For this review, take the finished solid that the model builds, in its own axes (mm). A direction names the side the tool comes from. Coordinates: 2 decimals unless noted, no trailing zeros. Loops run counter-clockwise (first coordinate to the right, second up) from the corner with the lowest first, then second, coordinate; pieces in that order, holes last. Notation, with made-up numbers: (7, 34) - (62, 34) arc R14 ccw to (62, 49) - close; hole circle Ø7 at (52.5, -26.5). An arc over 180 degrees is marked (long way). Answer as a JSON object with one key per item and string values. Group by question number.
Item 1: We need section B-B (z = 0). Give the boundary of the cut face in (x, y) (1 decimal), then the cut area to 3 significant figures.
Item 2: We need section C-C (y = 15.5). Give the boundary of the cut face in (x, z).
Item 3: To check wall thickness, follow line 1 (Y direction, x = 0, z = 5.4); line 2 (Z direction, x = -2.75, y = 20.75); line 3 (Y direction, x = 0.5, z = -5). State the ranges of each line that lie inside material, in increasing order.
Item 4: Tool access review of faces 1 (the flat face through (0, 6, -4.064)), 2 (the flat face through (3.086, 18, 0)), 3 (the flat face through (0, 18, -3.086)), 4 (the flat face through (-3.086, 18, 0)): name each direction out of +Z, -Z, +X, -X, +Y, -Y from which nothing blocks a thin tool from reaching the whole face with its end or side.
Item 5: Mouldability with a two-part tool opening along Z and no side actions: class faces 5 (the flat face through (0, 18, 3.086)), 6 (the flat face through (0, 6, 4.064)), 7 (the flat face through (0, 21.387, 0)), 8 (the conical face through (2.81, 21.23, -2.8)) as released by +Z, released by -Z, zero draft, split by the parting line, or undercut.
Item 6: We need section D-D (y = 10). Give the boundary of the cut face in (x, z), then the cut area to 3 significant figures.
Item 7: We need section A-A (x = 0). Give the boundary of the cut face in (y, z) (1 decimal), then the cut area to 3 significant figures.
Item 8: Clearance check with flat-ended pins moving along their axes: pin 1 (3 mm diameter, centred on x = -4, z = -1.5, fed in from -Y) (3 decimals); pin 2 (4 mm diameter, centred on x = -3.5, y = 7.5, fed in from +Z); pin 3 (1.9 mm diameter, centred on x = -0.5, y = 16.5, fed in from +Z). State where each tip first meets the part, or that it passes through.
from build123d import *

# Parameters (mm, degrees)
BASE_R                  = 6.9215
BASE_EXTRUDE_DEPTH      = 13.716
MALEDRIVE_R             = 6.0579
DRIVE_EXTRUDE_DEPTH     = 7.6708
SQDRIVE_SK_OUTSIDE_W    = 21.642
SQDRIVE_SK_OUTSIDE_H    = 21.642
SQDRIVE_SK_OUTSIDE_W_2  = 6.1722
SQDRIVE_SK_OUTSIDE_H_2  = 6.1722
DRIVE_SQCUT_DEPTH       = 7.6708
BASE_FILLET_TOP_R       = 0.762
PROFILE1_CUT_DEPTH      = 24.520406857
PROFILE1_CUT_DEPTH_BACK = 24.520406857
PROFILE1_CUTSK_W        = 8.128
PROFILE1_CUTSK_H        = 9.525
PROFILE2_CUT_DEPTH      = 24.520406857
PROFILE2_CUT_DEPTH_BACK = 24.520406857
PIN_CUT_DEPTH           = 24.520406916
PIN_CUT_DEPTH_BACK      = 24.520406916
PIN_CUTSK_R             = 1.778


with BuildPart() as part:
    # Base → Base-Extrude (new body)
    with BuildSketch(Plane(origin=(0, 0, 0), x_dir=(1, 0, 0), z_dir=(0, 1, 0))):
        with Locations(Location((0, 0, 0), (0, 0, 270))):
            Circle(BASE_R)
    extrude(amount=BASE_EXTRUDE_DEPTH)

    # MaleDrive → Drive-Extrude (add)
    with BuildSketch(Plane(origin=(0, 13.716, 0), x_dir=(1, 0, 0), z_dir=(0, 1, 0))):
        with Locations(Location((0, 0, 0), (0, 0, 270))):
            Circle(MALEDRIVE_R)
    extrude(amount=DRIVE_EXTRUDE_DEPTH)

    # Drive-ChamCut → DriveEnd-Chamfer (revolve, cut)
    with BuildSketch(Plane.XY, mode=Mode.PRIVATE) as driveend_chamfer_sk:
        Polygon((-3.81, 21.3868), (-5.4229, 19.7739), (-5.4229, 21.3868), align=None)
    revolve(driveend_chamfer_sk.sketch.rotate(Axis((0, 0, 0), (0, 1, 0)), 270), axis=Axis((0, 0, 0), (0, 1, 0)), mode=Mode.SUBTRACT)

    # SQDrive-Sk outside → Drive-SQCut (cut)
    with BuildSketch(Plane(origin=(0, 21.3868, 0), x_dir=(-1, 0, 0), z_dir=(0, 1, 0))):
        Rectangle(SQDRIVE_SK_OUTSIDE_W, SQDRIVE_SK_OUTSIDE_H)
        Rectangle(SQDRIVE_SK_OUTSIDE_W_2, SQDRIVE_SK_OUTSIDE_H_2, mode=Mode.SUBTRACT)
    extrude(amount=-DRIVE_SQCUT_DEPTH, mode=Mode.SUBTRACT)

    # Base-Fillet_Top
    base_fillet_top_edges = [part.edges().sort_by_distance(p)[0] for p in [
        (0, 13.716, -6.9215),
    ]]
    fillet(base_fillet_top_edges, radius=BASE_FILLET_TOP_R)

    # Profile1-CutSk → Profile1-Cut (cut, two sides: drawn at the far end of the back side and taken through both)
    with BuildSketch(Plane(origin=(0, 0, 0), x_dir=(0, 0, -1), z_dir=(1, 0, 0)).offset(-PROFILE1_CUT_DEPTH_BACK)):
        with Locations((0, 4.7625)):
            Rectangle(PROFILE1_CUTSK_W, PROFILE1_CUTSK_H)
    extrude(amount=PROFILE1_CUT_DEPTH + PROFILE1_CUT_DEPTH_BACK, mode=Mode.SUBTRACT)

    # Profile2-CutSk → Profile2-Cut (cut, two sides: drawn at the far end of the back side and taken through both)
    with BuildSketch(Plane.XY.offset(-PROFILE2_CUT_DEPTH_BACK)):
        with BuildLine():
            Line((53.381392937, 9.525), (6.9215, 9.525))
            Line((6.9215, 9.525), (4.953, 9.525))
            Line((4.953, 9.525), (2.674532127, 1.985721643))
            ThreePointArc((2.674532127, 1.985721643), (0, 0), (-2.674532127, 1.985721643))
            Line((-2.674532127, 1.985721643), (-4.953, 9.525))
            Line((-4.953, 9.525), (-6.9215, 9.525))
            Line((-6.9215, 9.525), (-53.381392937, 9.525))
            Line((-53.381392937, 9.525), (-53.381392937, -83.394785874))
            Line((-53.381392937, -83.394785874), (53.381392937, -83.394785874))
            Line((53.381392937, -83.394785874), (53.381392937, 9.525))
        make_face()
    extrude(amount=PROFILE2_CUT_DEPTH + PROFILE2_CUT_DEPTH_BACK, mode=Mode.SUBTRACT)

    # Pin-CutSk → Pin-Cut (cut, two sides: drawn at the far end of the back side and taken through both)
    with BuildSketch(Plane.XY.offset(-PIN_CUT_DEPTH_BACK)):
        with Locations(Location((0, 2.794, 0), (0, 0, 90))):
            Circle(PIN_CUTSK_R)
    extrude(amount=PIN_CUT_DEPTH + PIN_CUT_DEPTH_BACK, mode=Mode.SUBTRACT)


solid = part.part
Check sheet entries:
{
 "1": {"outline": "(-6.9, 9.5) - (6.9, 9.5) - (6.9, 13) arc R0.8 ccw to (6.2, 13.7) - (3.1, 13.7) - (3.1, 21.4) - (-3.1, 21.4) - (-3.1, 13.7) - (-6.2, 13.7) arc R0.8 ccw to (-6.9, 13) - close", "area": "105 mm2"},
 "2": {"outline": "(-3.09, -3.09) - (3.09, -3.09) - (3.09, 3.09) - (-3.09, 3.09) - close"},
 "3": {"line 1": "y = 0 to 1.02, 4.57 to 13.72", "line 2": "z = -3.09 to 3.09", "line 3": "y = 0.05 to 1.09, 4.5 to 13.72"},
 "4": {"face 1": "+X, -X, -Y", "face 2": "+Z, -Z, +X, +Y", "face 3": "-Z, +X, -X, +Y", "face 4": "+Z, -Z, -X, +Y"},
 "5": {"face 5": "released by +Z", "face 6": "undercut", "face 7": "zero draft", "face 8": "released by -Z"},
 "6": {"outline": "circle Ø13.84 at (0, 0)", "area": "151 mm2"},
 "7": {"outline": "(0, -6.9) - (1, -6.9) - (1, -4.1) - (0, -4.1) - close; (0, 4.1) - (1, 4.1) - (1, 6.9) - (0, 6.9) - close; (4.6, -6.9) - (13, -6.9) arc R0.8 ccw to (13.7, -6.2) - (13.7, -3.1) - (21.4, -3.1) - (21.4, 3.1) - (13.7, 3.1) - (13.7, 6.2) arc R0.8 ccw to (13, 6.9) - (4.6, 6.9) - (4.6, 4.1) - (9.5, 4.1) - (9.5, -4.1) - (4.6, -4.1) - close", "area": "139 mm2"},
 "8": {"pin 1": "stops at y = 9.525", "pin 2": "stops at z = 6.76", "pin 3": "stops at z = 3.09"}
}
